Verification items for the finished model (mm, model axes). Face numbers are marked on the shaded views. Give positions to 0.01 mm unless a question says otherwise; leave off trailing zeros. Order: outer loops, then holes, each group sorted by start corner. A loop starts at its lowest first (then second) coordinate and runs counter-clockwise, first axis right, second up.
from build123d import *

# Parameters (mm, degrees)
SKETCH1_W           = 15
SKETCH1_H           = 9
BOSS_EXTRUDE1_DEPTH = 9
SKETCH2_R           = 1.5875
CUT_EXTRUDE1_DEPTH  = 13.549900398
SKETCH3_R           = 1.5875
CUT_EXTRUDE2_DEPTH  = 15.773286703


with BuildPart() as part:
    # Sketch1 → Boss-Extrude1 (new body)
    with BuildSketch(Plane(origin=(0, 0, 0), x_dir=(1, 0, 0), z_dir=(0, 1, 0))):
        Rectangle(SKETCH1_W, SKETCH1_H)
    extrude(amount=BOSS_EXTRUDE1_DEPTH)

    # Sketch2 → Cut-Extrude1 (cut, through all)
    with BuildSketch(Plane(origin=(0, 9, 0), x_dir=(1, 0, 0), z_dir=(0, 1, 0))):
        with Locations(Location((0, 0, 0), (0, 0, 270))):
            Circle(SKETCH2_R)
    extrude(amount=-CUT_EXTRUDE1_DEPTH, mode=Mode.SUBTRACT)

    # Sketch3 → Cut-Extrude2 (cut, through all)
    with BuildSketch(Plane.XY.offset(4.5)):
        with Locations((-3.75, 4.5)):
            Circle(SKETCH3_R)
        with Locations(Location((3.75, 4.5, 0), (0, 0, 180))):
            Circle(SKETCH3_R)
    extrude(amount=-CUT_EXTRUDE2_DEPTH, mode=Mode.SUBTRACT)


solid = part.part
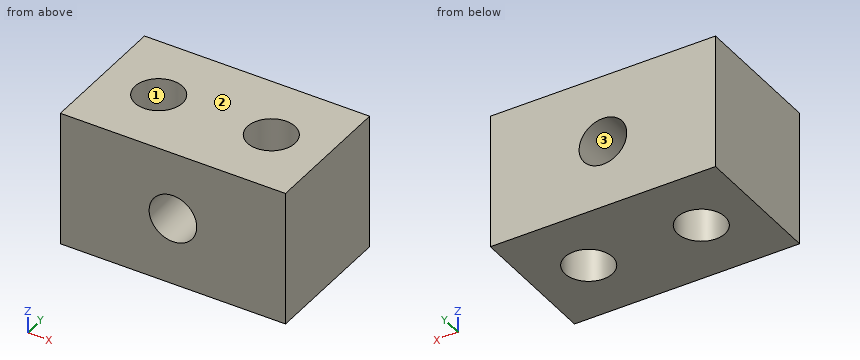
(1) Go/stop test with a flat-tipped pin: pin 1 (1.9 mm diameter, centred on x = -3.75, y = 4.5, fed in from +Z). Record where the tip stops, or that it passes through.
Solved:
pin 1: passes through
(2) Section check C-C, the plane x = 3.75. Enter the section's corners in (y, z).
Solved:
outline: (0, -4.5) - (2.91, -4.5) - (2.91, 4.5) - (0, 4.5) - close; (6.09, -4.5) - (9, -4.5) - (9, 4.5) - (6.09, 4.5) - close
(3) Scan lines: line 1 (X direction, y = 3.75, z = 0); line 2 (Y direction, x = 3.75, z = -0.75); line 3 (X direction, y = 5.5, z = 1). Record each from-to range of solid material in increasing order.
Solved:
line 1: x = -7.5 to -5.15, -2.35 to -1.59, 1.59 to 2.35, 5.15 to 7.5
line 2: y = 0 to 2.91, 6.09 to 9
line 3: x = -7.5 to -4.98, -2.52 to -1.23, 1.23 to 2.52, 4.98 to 7.5
(4) Release check for a two-part mould opening along Z. For the marked faces 1, 2 and 3 record: pulls with the +Z half, pulls with the -Z half, needs draft (parallel to the pull), parting line crosses it, or undercut.
Solved:
face 1: needs draft
face 2: pulls with the +Z half
face 3: undercut
(5) Section check A-A, the plane z = 0. Give the number of separate pieces and of enclosed holes in the cut face, then the cut area to 3 significant figures.
Solved:
separate pieces: 2
enclosed holes: 2
area: 90.6 mm2
(6) Section check B-B, the plane y = 4.5. Enter the section's corners in (x, z) (1 decimal), then the cut area to 3 significant figures.
Solved:
outline: (-7.5, -4.5) - (-5.3, -4.5) - (-5.3, 4.5) - (-7.5, 4.5) - close; (-2.2, -4.5) - (2.2, -4.5) - (2.2, 4.5) - (-2.2, 4.5) - close; (5.3, -4.5) - (7.5, -4.5) - (7.5, 4.5) - (5.3, 4.5) - close; hole circle Ø3.2 at (0, 0)
area: 69.9 mm2
